Can you work these out from the model? Positions are in its coordinate system, mm. Round coordinates to 2 decimals unless told otherwise and drop trailing zeros. Loops run counter-clockwise (first coordinate to the right, second up) from the corner with the lowest first, then second, coordinate; pieces in that order, holes last.
(1) I want a section at B-B on y = 34.5. Write out the boundary of the cut face in (x, z).
(2) If I drill on line 1 along Z through (x, y) = (103, -3); line 2 along Z through (x, y) = (126.5, 90.5); line 3 along Y through (x, z) = (77.5, -142), over which ranges is the centre line in solid material (lowest first)?
(3) Thinking about a two-plate mould opening in Y: for faces 1 (the face through (8.86, -5.7, -179.62)), 2 (the face through (66, -6, -178.054)), 3 (the face through (66, -11.303, -180)), which applies, released by +Y, released by -Y, zero draft, split by the parting line, or undercut?
(4) I want a section at A-A on x = 81. Write out the boundary of the cut face in (y, z).
(5) Will these pins go through, and if not, where does the flat tip stop? pin 1 Ø10 at (x, y) = (37.5, 60.5) entering from -Z; pin 2 Ø5 at (x, y) = (7.874, -7.239) entering from +Z; pin 3 Ø2 at (x, y) = (125.476, -7.239) entering from -Z; pin 4 Ø6 at (x, y) = (81, 36.5) entering from -Z.
from build123d import *

# Parameters (mm, degrees)
BOSS_EXTRUDE1_DEPTH = 133.35
CUT_EXTRUDE1_DEPTH  = 134.35
SKETCH3_W           = 133.35
SKETCH3_H           = 3.175
BOSS_EXTRUDE2_DEPTH = 11.303
SKETCH4_R           = 1.8288
CUT_EXTRUDE2_DEPTH  = 4.175


with BuildPart() as part:
    # Sketch1 → Boss-Extrude1 (new body)
    with BuildSketch(Plane(origin=(0, 0, 0), x_dir=(0, 0, -1), z_dir=(1, 0, 0))):
        with BuildLine():
            Line((0, 178.054), (0, 181.229))
            ThreePointArc((0, 181.229), (128.148254848, 128.148254848), (181.229, 0))
            Line((181.229, 0), (178.054, 0))
            ThreePointArc((178.054, 0), (125.903190817, 125.903190817), (0, 178.054))
        make_face()
    extrude(amount=BOSS_EXTRUDE1_DEPTH)

    # Sketch2 → Cut-Extrude1 (cut, through all)
    with BuildSketch(Plane(origin=(133.35, 0, 0), x_dir=(0, 0, -1), z_dir=(1, 0, 0))):
        with BuildLine():
            Line((114.450905055, 136.397277275), (116.491755716, 138.829468382))
            ThreePointArc((116.491755716, 138.829468382), (61.983968555, 170.299553972), (0, 181.229))
            Line((0, 181.229), (0, 178.054))
            ThreePointArc((0, 178.054), (60.8980546, 167.316029901), (114.450905055, 136.397277275))
        make_face()
    extrude(amount=-CUT_EXTRUDE1_DEPTH, mode=Mode.SUBTRACT)

    # Sketch3 → Boss-Extrude2 (add)
    with BuildSketch(Plane.XZ):
        with Locations((66.675, -179.6415)):
            Rectangle(SKETCH3_W, SKETCH3_H)
    extrude(amount=BOSS_EXTRUDE2_DEPTH)

    # Sketch4 → Cut-Extrude2 (cut, through all)
    with BuildSketch(Plane.XY.offset(-178.054)):
        with Locations((7.874, -7.239)):
            Circle(SKETCH4_R)
        with Locations((58.801, -7.239)):
            Circle(SKETCH4_R)
        with Locations((74.549, -7.239)):
            Circle(SKETCH4_R)
        with Locations((125.476, -7.239)):
            Circle(SKETCH4_R)
    extrude(amount=-CUT_EXTRUDE2_DEPTH, mode=Mode.SUBTRACT)


solid = part.part
Filled sheet:
1. outline: (0, -177.91) - (133.35, -177.91) - (133.35, -174.68) - (0, -174.68) - close
2. line 1: z = -181.23 to -178.05
2. line 2: z = -157.01 to -153.34
2. line 3: y = 107.42 to 112.61
3. face 1: undercut
3. face 2: zero draft
3. face 3: released by -Y
4. outline: (-11.3, -181.23) - (0, -181.23) arc R181.23 ccw to (138.83, -116.49) - (136.4, -114.45) arc R178.05 cw to (0, -178.05) - (-11.3, -178.05) - close
5. pin 1: stops at z = -172.52
5. pin 2: stops at z = -178.05
5. pin 3: passes through
5. pin 4: stops at z = -178.11
